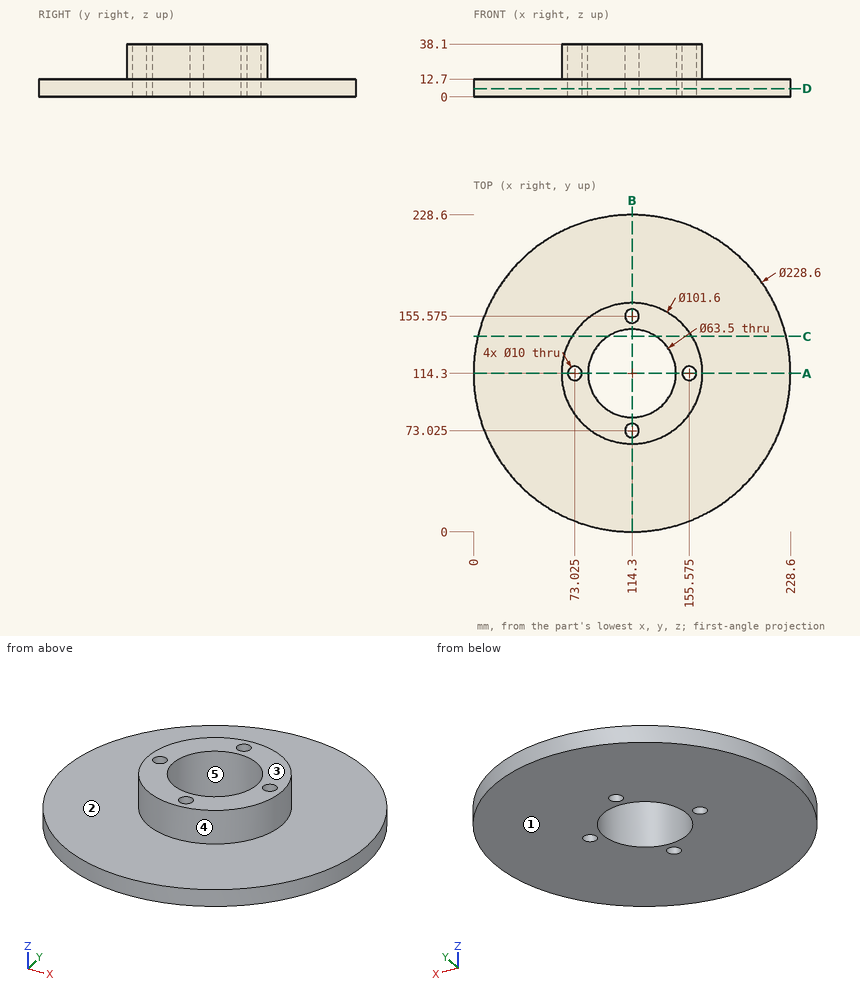
Input: dimensioned drawing with shaded views. Units: mm. Origin: part minimum x, y, z. A direction names the side the tool comes from. Coordinates: 2 decimals unless noted, no trailing zeros. Loops run counter-clockwise (first coordinate to the right, second up) from the corner with the lowest first, then second, coordinate; pieces in that order, holes last. Notation, with made-up numbers: (-26, -26.5) -> (7, -26.5) arc R20 cw to (7, -7.5) -> close; hole circle Ø6 at (27.25, -6.5). An arc over 180 degrees is marked (long way). Use a Markdown table: item, result. Add a question column.
(1) Section query A-A, the plane y = 114.3. Return loops of the section in (x, z) (3 decimals), plus the area to 3 significant figures.
(2) Section query C-C, the plane y = 141. Return loops of the section in (x, z).
(3) Access query for the marked faces 1 and 2. Directions: +Z, -Z, +X, -X, +Y, -Y. A direction counts if a zero-diameter tool reaches every point of the face in a straight line with its end or side. Return the directions, or none.
(4) Section query D-D, the plane z = 6. Return loops of the section in (x, y) (3 decimals).
(5) Line query: line 1 along Y through (x, z) = (114.3, 18.5) (3 decimals); line 2 along Y through (x, z) = (115, 27); line 3 along Z through (x, y) = (18.5, 120). Output: solid intervals per line, ascending.
(6) Mould query, pull axis X, two halves, no side actions, for the marked faces 3, 4 and 5. Classes: pulls with the +X half, pulls with the -X half, needs draft (parallel to the pull), parting line crosses it, or undercut.
(7) Pin query (flat end, axial travel): pin 1 Ø1 at (y, z) = (149.5, 16) entering from -X; pin 2 Ø13 at (x, y) = (114.3, 155.575) entering from +Z; pin 3 Ø6 at (x, z) = (156.5, 29.5) entering from +Y; pin 4 Ø6 at (x, z) = (56, 14) entering from -Y. Return the tip coordinate at first contact, or that it passes through.
Answer:
| question | item | result |
|---|---|---|
| 1 | outline | (0, 0) -> (68.025, 0) -> (68.025, 38.1) -> (63.5, 38.1) -> (63.5, 12.7) -> (0, 12.7) -> close; (78.025, 0) -> (82.55, 0) -> (82.55, 38.1) -> (78.025, 38.1) -> close; (146.05, 0) -> (150.575, 0) -> (150.575, 38.1) -> (146.05, 38.1) -> close; (160.575, 0) -> (228.6, 0) -> (228.6, 12.7) -> (165.1, 12.7) -> (165.1, 38.1) -> (160.575, 38.1) -> close |
| 1 | area | 2,300 mm^2 |
| 2 | outline | (3.16, 0) -> (97.12, 0) -> (97.12, 38.1) -> (71.08, 38.1) -> (71.08, 12.7) -> (3.16, 12.7) -> close; (131.48, 0) -> (225.44, 0) -> (225.44, 12.7) -> (157.52, 12.7) -> (157.52, 38.1) -> (131.48, 38.1) -> close |
| 3 | face 1 | -Z, +X, -X, +Y, -Y |
| 3 | face 2 | +Z |
| 4 | outline | circle Ø228.6 at (114.3, 114.3); hole circle Ø10 at (73.025, 114.3); hole circle Ø63.5 at (114.3, 114.3); hole circle Ø10 at (114.3, 73.025); hole circle Ø10 at (114.3, 155.575); hole circle Ø10 at (155.575, 114.3) |
| 5 | line 1 | y = 63.5 to 68.025, 78.025 to 82.55, 146.05 to 150.575, 160.575 to 165.1 |
| 5 | line 2 | y = 63.5 to 68.07, 77.98 to 82.56, 146.04 to 150.62, 160.53 to 165.1 |
| 5 | line 3 | z = 0 to 12.7 |
| 6 | face 3 | needs draft |
| 6 | face 4 | parting line crosses it |
| 6 | face 5 | undercut |
| 7 | pin 1 | stops at x = 77.2 |
| 7 | pin 2 | stops at z = 38.1 |
| 7 | pin 3 | stops at y = 146.61 |
| 7 | pin 4 | stops at y = 14.43 |
